Can you work these out from the model? Positions are in its coordinate system, mm. Round coordinates to 2 decimals unless told otherwise and drop trailing zeros. Write each loop counter-clockwise with the first axis right and the second up, starting at its lowest first coordinate (ties: lowest second). Pieces come first, ordered by that corner, then holes. Notation, with made-up numbers: (14.25, 73.5) -> (36.25, 73.5) arc R23 cw to (36.25, 104.5) -> close; hole circle Ø10 at (89.5, 49.5). An arc over 180 degrees is marked (long way). Use CSV: the item, a comma, the result in double quotes.
```python
from build123d import *

# Parameters (mm, degrees)
SKETCH1_R                                         = 3.175
SKETCH1_R_2                                       = 4
BOSS_EXTRUDE1_DEPTH                               = 3.175
CSK_FOR_6_FLAT_HEAD_MACHINE_SCREW_100_D           = 3.6576
CSK_FOR_6_FLAT_HEAD_MACHINE_SCREW_100_DEPTH       = 8
CSK_FOR_6_FLAT_HEAD_MACHINE_SCREW_100_CSINK_D     = 7.0866
CSK_FOR_6_FLAT_HEAD_MACHINE_SCREW_100_CSINK_ANGLE = 100
CSK_FOR_6_FLAT_HEAD_MACHINE_SCREW_100_TIP         = 1.0988539


with BuildPart() as part:
    # Sketch1 → Boss-Extrude1 (new body)
    with BuildSketch(Plane.XY):
        with BuildLine():
            Line((-55, -38.509768834), (-22.199103684, -38.509768834))
            Line((-22.199103684, -38.509768834), (4.467936384, -35.116912513))
            ThreePointArc((4.467936384, -35.116912513), (32.876567079, -13.125979473), (27.425045484, 22.383629737))
            Line((27.425045484, 22.383629737), (10.098875196, 43.612135293))
            ThreePointArc((10.098875196, 43.612135293), (9.013562327, 44.539147516), (7.671865627, 45.026082472))
            ThreePointArc((7.671865627, 45.026082472), (0, 45.675), (-7.671865627, 45.026082472))
            Line((-7.671865627, 45.026082472), (-55, 32.491174512))
            Line((-55, 32.491174512), (-55, -38.509768834))
        make_face()
        with Locations((0, 39.175)):
            Circle(SKETCH1_R, mode=Mode.SUBTRACT)
        Circle(SKETCH1_R_2, mode=Mode.SUBTRACT)
    extrude(amount=-BOSS_EXTRUDE1_DEPTH)

    # CSK for #6 Flat Head Machine Screw (100)1
    with Locations(Plane(origin=(0, 0, -3.175), x_dir=(-1, 0, 0), z_dir=(0, 0, -1))):
        with Locations((50, 26), (39, 0), (50, -30), (25, 30), (25, -30)):
            CounterSinkHole(CSK_FOR_6_FLAT_HEAD_MACHINE_SCREW_100_D / 2, CSK_FOR_6_FLAT_HEAD_MACHINE_SCREW_100_CSINK_D / 2, depth=CSK_FOR_6_FLAT_HEAD_MACHINE_SCREW_100_DEPTH, counter_sink_angle=CSK_FOR_6_FLAT_HEAD_MACHINE_SCREW_100_CSINK_ANGLE)
            with Locations((0, 0, -(CSK_FOR_6_FLAT_HEAD_MACHINE_SCREW_100_DEPTH + CSK_FOR_6_FLAT_HEAD_MACHINE_SCREW_100_TIP / 2))):  # 118° drill point
                Cone(0, CSK_FOR_6_FLAT_HEAD_MACHINE_SCREW_100_D / 2, CSK_FOR_6_FLAT_HEAD_MACHINE_SCREW_100_TIP, mode=Mode.SUBTRACT)


solid = part.part
```
Q1. Please list where these lines run through material, in increasing order: probe 1 along Y at (x, z) = (-25, -0.6); probe 2 along Y at (x, z) = (-50, -0.7); probe 3 along X at (y, z) = (-28.5, -2.4).
Resolved:
probe 1,"y = -38.51 to -31.83, -28.17 to 28.17, 31.83 to 40.44"
probe 2,"y = -38.51 to -31.83, -28.17 to 24.17, 27.83 to 33.82"
probe 3,"x = -55 to -52.15, -47.85 to -27.15, -22.85 to 21"
Q2. Suppose I cut it at C-C (z = -1). Write out the boundary of the cut face in (x, y) (3 decimals).
Resolved:
outline,"(-55, -38.51) -> (-22.199, -38.51) -> (4.468, -35.117) arc R35.4 ccw to (27.425, 22.384) -> (10.099, 43.612) arc R4 ccw to (7.672, 45.026) arc R45.675 ccw to (-7.672, 45.026) -> (-55, 32.491) -> close; hole circle Ø3.658 at (-50, -30); hole circle Ø3.658 at (-50, 26); hole circle Ø3.658 at (-39, 0); hole circle Ø3.658 at (-25, -30); hole circle Ø3.658 at (-25, 30); hole circle Ø8 at (0, 0); hole circle Ø6.35 at (0, 39.175)"
Q3. Suppose I cut it at B-B (x = -25). Write out the boundary of the cut face in (y, z) (3 decimals).
Resolved:
outline,"(-38.51, -3.175) -> (-33.543, -3.175) -> (-31.829, -1.736) -> (-31.829, 0) -> (-38.51, 0) -> close; (-28.171, -1.736) -> (-26.457, -3.175) -> (26.457, -3.175) -> (28.171, -1.736) -> (28.171, 0) -> (-28.171, 0) -> close; (31.829, -1.736) -> (33.543, -3.175) -> (40.437, -3.175) -> (40.437, 0) -> (31.829, 0) -> close"
Q4. If we mould it in two halves opening along Y, with no side actions, what happens to faces 1 (the face through (-55, -3, -2)), 2 (the face through (-37.256, 0.549, -0.856)), 3 (the face through (-0.867, -3.905, -1.565)), 4 (the face through (9.03, 44.53, -1.57))? For each: released by +Y, released by -Y, zero draft, split by the parting line, or undercut.
Resolved:
face 1,"zero draft"
face 2,"undercut"
face 3,"undercut"
face 4,"released by +Y"
Q5. Suppose I cut it at D-D (x = -39). Write out the boundary of the cut face in (y, z) (3 decimals), and give its area (3 significant figures).
Resolved:
outline,"(-38.51, -3.175) -> (-3.543, -3.175) -> (-1.829, -1.736) -> (-1.829, 0) -> (-38.51, 0) -> close; (1.829, -1.736) -> (3.543, -3.175) -> (36.729, -3.175) -> (36.729, 0) -> (1.829, 0) -> close"
area,"225 mm^2"
Q6. Will these pins go through, and if not, where does the flat tip stop? P1, Ø5, axis at x = -50, y = 26, coming from the +Z side; P2, Ø5, axis at x = -25, y = 30, coming from the -Z side; P3, Ø6, axis at x = -25, y = -30, coming from the -Z side; P4, Ø1, axis at x = 20.5, z = -2.5, coming from the -Y side.
Resolved:
P1,"stops at z = 0"
P2,"stops at z = -2.3"
P3,"stops at z = -2.72"
P4,"stops at y = -29.21"
Q7. Suppose I cut it at A-A (y = 0). Write out the boundary of the cut face in (x, z) (3 decimals).
Resolved:
outline,"(-55, -3.175) -> (-42.543, -3.175) -> (-40.829, -1.736) -> (-40.829, 0) -> (-55, 0) -> close; (-37.171, -1.736) -> (-35.457, -3.175) -> (-4, -3.175) -> (-4, 0) -> (-37.171, 0) -> close; (4, -3.175) -> (35.4, -3.175) -> (35.4, 0) -> (4, 0) -> close"
